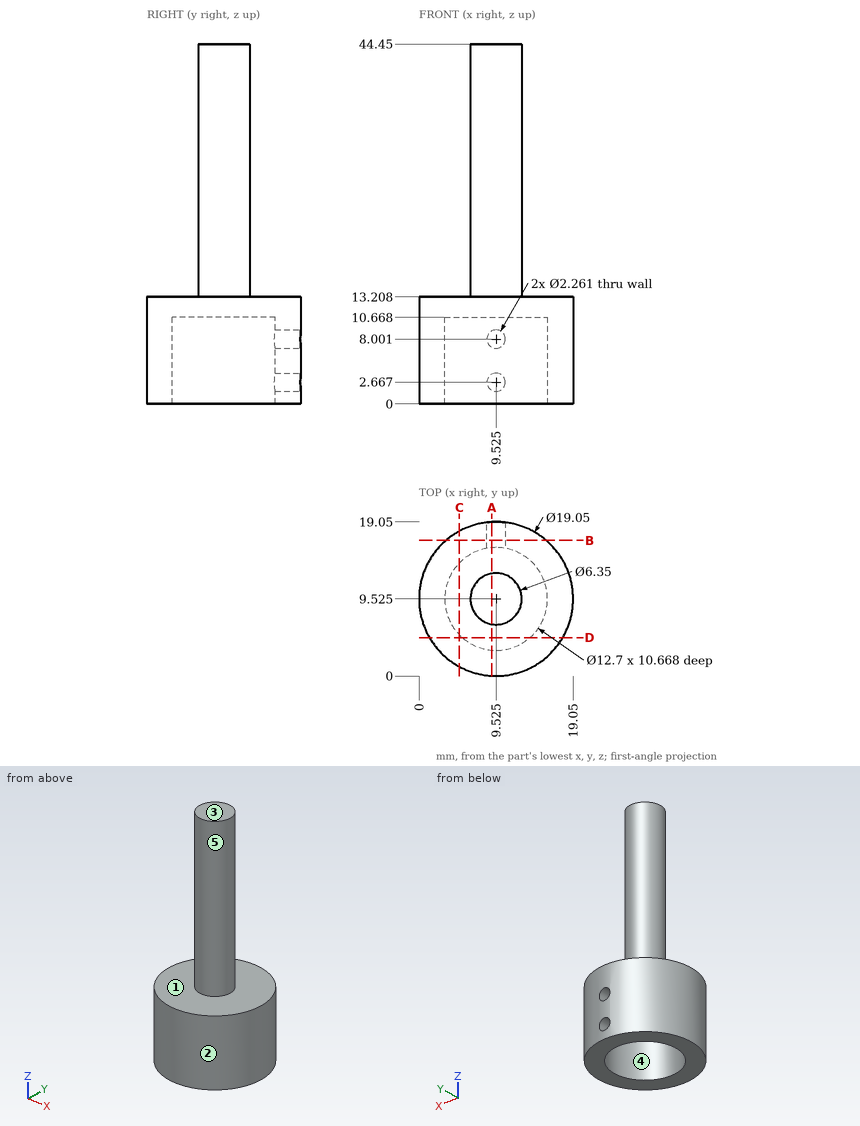
Study the drawing (mm; zero at the part's minimum x, y, z) and answer. A direction names the side the tool comes from. Round coordinates to 2 decimals unless told otherwise and drop trailing zeros. Loops run counter-clockwise (first coordinate to the right, second up) from the corner with the lowest first, then second, coordinate; pieces in that order, holes last.
Q1. Section C-C, the plane x = 5 is taken. Determine the outline of the cut face in (y, z), then the cut area to 3 significant figures.
Q2. Section A-A, the plane x = 9 is taken. Count the separate pieces of the cut face and the enclosed holes in it, then the cut area to 3 significant figures.
Q3. Section D-D, the plane y = 4.75 is taken. Determine the outline of the cut face in (x, z), then the cut area to 3 significant figures.
Q4. Section B-B, the plane y = 16.75 is taken. Determine the outline of the cut face in (x, z) (1 decimal), then the cut area to 3 significant figures.
Q5. Which of the six approach directions +Z, -Z, +X, -X, +Y, -Y give full straight-line access (tool end or side, diameter ignored) to the marked faces 1 and 2?
Q6. Given pin 1 Ø3 at (x, y) = (2.5, 6) entering from +Z; pin 2 Ø3.5 at (x, z) = (9.525, 2.667) entering from +Y; pin 3 Ø5 at (y, z) = (9.5, 32.5) entering from -X; pin 4 Ø7.5 at (x, y) = (9.525, 9.525) entering from -Z, each flat-ended and moving along its own axis, determine where each tip first touches the part or whether it passes through.
Q7. Find the intervals of material crossed by line 1 (X direction, y = 9.25, z = 8); line 2 (Y direction, x = 9.75, z = 30); line 3 (Z direction, x = 16.25, y = 14), in increasing order.
Q8. For a pull along Y with two mould halves and no side action, classify the marked faces 3, 4 and 5 as released by +Y, released by -Y, zero draft, split by the parting line, or undercut.
Completed:
1. outline: (1.14, 0) - (5.07, 0) - (5.07, 10.67) - (13.98, 10.67) - (13.98, 0) - (17.91, 0) - (17.91, 13.21) - (1.14, 13.21) - close
1. area: 126 mm2
2. separate pieces: 3
2. enclosed holes: 0
2. area: 299 mm2
3. outline: (1.28, 0) - (5.34, 0) - (5.34, 10.67) - (13.71, 10.67) - (13.71, 0) - (17.77, 0) - (17.77, 13.21) - (1.28, 13.21) - close
3. area: 128 mm2
4. outline: (3.3, 0) - (15.7, 0) - (15.7, 13.2) - (3.3, 13.2) - close; hole circle Ø2.3 at (9.5, 2.7); hole circle Ø2.3 at (9.5, 8)
4. area: 156 mm2
5. face 1: +Z
5. face 2: +Z, -Z
6. pin 1: stops at z = 13.21
6. pin 2: stops at y = 19.05
6. pin 3: stops at x = 6.35
6. pin 4: stops at z = 10.67
7. line 1: x = 0 to 3.18, 15.87 to 19.05
7. line 2: y = 6.36 to 12.69
7. line 3: z = 0 to 13.21
8. face 3: zero draft
8. face 4: undercut
8. face 5: split by the parting line
